Build history of the part. All positions in model axes, mm. A direction names the side the tool comes from. Round coordinates to 2 decimals unless told otherwise and drop trailing zeros. Loops run counter-clockwise (first coordinate to the right, second up) from the corner with the lowest first, then second, coordinate; pieces in that order, holes last. Notation, with made-up numbers: (74, 62.5) - (119, 62.5) arc R18 cw to (119, 94.5) - close; hole circle Ø8 at (10.25, 89). An arc over 180 degrees is marked (long way). Answer as CSV lines item,"result". Start each with the question number.
```python
from build123d import *

# Parameters (mm, degrees)
F0_W     = 132.1772886384
F0_H     = 91.3944654167
F0_W_2   = 123.5
F0_H_2   = 82.5
F1_DEPTH = 45
F2_W     = 160
F2_H     = 110.3064134685
F3_DEPTH = 4.6
F4_W     = 26.40013583
F4_H     = 8.1236897111
F4_H_2   = 8.12
F5_DEPTH = 115
F6_W     = 4.7950819135
F6_H     = 44.0778695047
F7_DEPTH = 115
F8_W     = 5.5164026618
F8_H     = 13.8319674879
F9_DEPTH = 115


# Not quite as in the source:
# - the program builds the solid bodies; features that only make, move or delete a surface that nothing else refers to are left out


with BuildPart() as f1:
    # F0 (on Top) → F1 (new body)
    with BuildSketch(Plane.XY):
        with Locations((-0.5622557336, 4.6925004572)):
            Rectangle(F0_W, F0_H)
        with Locations((-0.8209000528, 5.0862303376)):
            Rectangle(F0_W_2, F0_H_2, mode=Mode.SUBTRACT)
    extrude(amount=F1_DEPTH)

    # F2 (on Top) → F3 (join)
    with BuildSketch(Plane.XY):
        with Locations((-1.752063632, 4.8872958869)):
            Rectangle(F2_W, F2_H)
    extrude(amount=-F3_DEPTH)

    # F4 (on face) → F5 (join)
    with BuildSketch(Plane(origin=(0, 0, -4.6), x_dir=(1, 0, 0), z_dir=(0, 0, -1))):
        with Locations((19.0718499944, 38.1715348911)):
            Rectangle(F4_W, F4_H)
        with Locations((19.0718499944, -48.4503099644)):
            Rectangle(F4_W, F4_H_2)
    extrude(amount=F5_DEPTH)

    # F6 (on face) + F4 (on face) → F7 (join)
    with BuildSketch(Plane(origin=(0, 0, -4.6), x_dir=(1, 0, 0), z_dir=(0, 0, -1))):
        with Locations((73.7704820931, 0.2766400576)):
            Rectangle(F6_W, F6_H)
    with BuildSketch(Plane(origin=(0, 0, -4.6), x_dir=(1, 0, 0), z_dir=(0, 0, -1))):
        with Locations((19.0718499944, 38.1715348911)):
            Rectangle(F4_W, F4_H)
        with Locations((19.0718499944, -48.4503099644)):
            Rectangle(F4_W, F4_H_2)
    extrude(amount=F7_DEPTH)

    # F8 (on face) → F9 (join)
    with BuildSketch(Plane(origin=(0, 0, -4.6), x_dir=(1, 0, 0), z_dir=(0, 0, -1))):
        with Locations((-74.8852601945, 6.915983744)):
            Rectangle(F8_W, F8_H)
    extrude(amount=F9_DEPTH)


solid = f1.part
```
Q1. Band-saw the part on D-D, the plane x = 14. List the corners of the cut face in (y, z).
Q2. Pin check, flat tips, straight feed: pin 1 Ø5 at (x, y) = (28, 28.5) entering from -Z; pin 2 Ø22 at (y, z) = (-9, -71) entering from -X; pin 3 Ø22.5 at (x, z) = (-19, 30) entering from +Y. Stop position of each tip, or through.
Q3. Band-saw the part on B-B, the plane z = 22.5. List the corners of the cut face in (x, y), then the cut area to 3 significant figures.
Q4. Two-plate mould, pull along X, no slides. Class faces 1 (the flat face through (-2, 6, 0)), 2 (the flat face through (65.526, 4, 22)), 3 (the flat face through (-66.651, 4, 22)), 4 (the flat face through (-1, 50.39, 22)): released by +X, released by -X, zero draft, split by the parting line, or undercut.
Q5. Band-saw the part on C-C, the plane y = 39. List the corners of the cut face in (x, z), then the cut area to 3 significant figures.
Q6. Tool access for faces 5 (the flat face through (-75, -13.832, -61)), 6 (the flat face through (19, 52.51, -61)), 7 (the flat face through (-2, 46.336, 22)), 8 (the flat face through (76.168, 0, -61)), 9 (the flat face through (-77.643, -7, -61)): list every direction of +Z, -Z, +X, -X, +Y, -Y with a clear straight run to the whole face (end or side of a thin tool).
Q7. Band-saw the part on A-A, the plane z = -100.5. List the corners of the cut face in (x, y), then the cut area to 3 significant figures.
Q8. Wall check: probe 1 along Y at (x, z) = (-48.5, 15); probe 2 along X at (y, z) = (-35.5, 5); probe 3 along Z at (x, y) = (-20.5, 30). Give the ranges that are in metal, low to high. Write a range as [from, to].
Reported:
1,outline,"(-50.27, -4.6) - (-42.23, -4.6) - (-42.23, -119.6) - (-34.11, -119.6) - (-34.11, -4.6) - (44.39, -4.6) - (44.39, -119.6) - (52.51, -119.6) - (52.51, -4.6) - (60.04, -4.6) - (60.04, 0) - (50.39, 0) - (50.39, 45) - (46.34, 45) - (46.34, 0) - (-36.16, 0) - (-36.16, 45) - (-41, 45) - (-41, 0) - (-50.27, 0) - close"
2,pin 1,"stops at z = -4.6"
2,pin 2,"stops at x = -77.64"
2,pin 3,"stops at y = 50.39"
3,outline,"(-66.65, -41) - (65.53, -41) - (65.53, 50.39) - (-66.65, 50.39) - close; hole (-62.57, -36.16) - (60.93, -36.16) - (60.93, 46.34) - (-62.57, 46.34) - close"
3,area,"1,890 mm2"
4,face 1,"undercut"
4,face 2,"released by +X"
4,face 3,"released by -X"
4,face 4,"zero draft"
5,outline,"(-81.75, -4.6) - (78.25, -4.6) - (78.25, 0) - (65.53, 0) - (65.53, 45) - (60.93, 45) - (60.93, 0) - (-62.57, 0) - (-62.57, 45) - (-66.65, 45) - (-66.65, 0) - (-81.75, 0) - close"
5,area,"1,130 mm2"
6,face 5,"-Z, -X, -Y"
6,face 6,"-Z, +X, -X, +Y"
6,face 7,"+Z"
6,face 8,"-Z, +X, +Y, -Y"
6,face 9,"-Z, -X, +Y, -Y"
7,outline,"(-77.64, -13.83) - (-72.13, -13.83) - (-72.13, 0) - (-77.64, 0) - close; (5.87, -42.23) - (32.27, -42.23) - (32.27, -34.11) - (5.87, -34.11) - close; (5.87, 44.39) - (32.27, 44.39) - (32.27, 52.51) - (5.87, 52.51) - close; (71.37, -22.32) - (76.17, -22.32) - (76.17, 21.76) - (71.37, 21.76) - close"
7,area,"716 mm2"
8,probe 1,"y = [-41, -36.16], [46.34, 50.39]"
8,probe 2,"x = [-66.65, -62.57], [60.93, 65.53]"
8,probe 3,"z = [-4.6, 0]"
